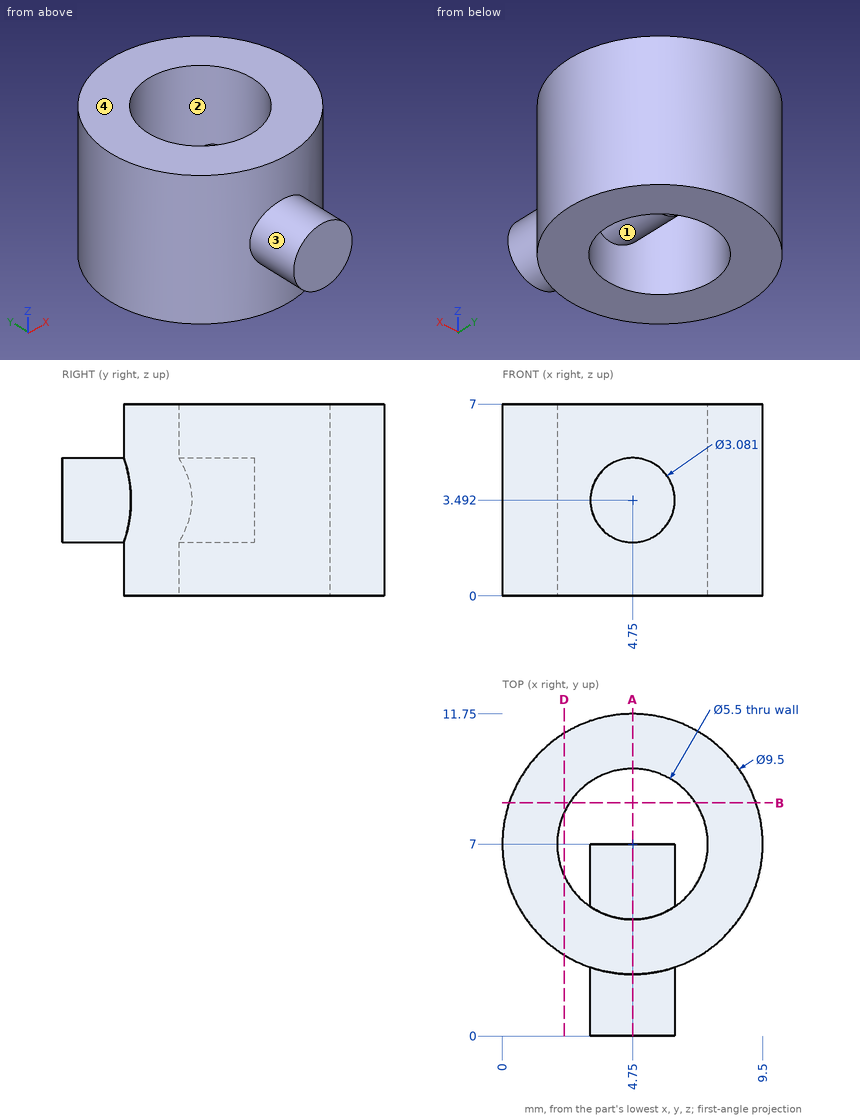
Answer from the drawing. Dimensions are ordinates in mm from the lowest x, y and z of the part. Coordinates: 2 decimals unless noted, no trailing zeros. Order: outer loops, then holes, each group sorted by start corner. A loop starts at its lowest first (then second) coordinate and runs counter-clockwise, first axis right, second up. Notation, with made-up numbers: (-32, 43.5) - (18, 43.5) arc R12 cw to (18, 52.5) - close; hole circle Ø10 at (52, 81.5). An arc over 180 degrees is marked (long way). Put each result on its own line as item: value. Start each with the question number.
1) Find section A-A (x = 4.75). Give the vertices of the cut face in (y, z).
2) Find the intervals of material crossed by line 1 (Y direction, x = 4.75, z = 2.25); line 2 (Y direction, x = 4.75, z = 1.5); line 3 (X direction, y = 6.25, z = 3.5) (1 decimal), in increasing order. Write a range as from..to.
3) Find section B-B (y = 8.5). Give the vertices of the cut face in (x, z) (1 decimal).
4) For a pull along X with two mould halves and no side action, classify the marked faces 1, 2, 3 and 4 as released by +X, released by -X, zero draft, split by the parting line, or undercut.
5) Find section D-D (x = 2.25). Give the vertices of the cut face in (y, z) (1 decimal).
6) A flat-ended cylindrical pin translates along its axis: pin 1 (3.5 mm diameter, centred on x = 4.75, y = 7, fed in from -Z). Find the tip coordinate at first contact, or state that the pin passes through.
Results list:
1. outline: (0, 1.95) - (2.25, 1.95) - (2.25, 0) - (4.25, 0) - (4.25, 1.95) - (7, 1.95) - (7, 5.03) - (4.25, 5.03) - (4.25, 7) - (2.25, 7) - (2.25, 5.03) - (0, 5.03) - close; (9.75, 0) - (11.75, 0) - (11.75, 7) - (9.75, 7) - close
2. line 1: y = 0..7, 9.75..11.75
2. line 2: y = 2.25..4.25, 9.75..11.75
2. line 3: x = 0.1..2.1, 3.2..6.3, 7.4..9.4
3. outline: (0.2, 0) - (2.4, 0) - (2.4, 7) - (0.2, 7) - close; (7.1, 0) - (9.3, 0) - (9.3, 7) - (7.1, 7) - close
4. face 1: undercut
4. face 2: undercut
4. face 3: split by the parting line
4. face 4: zero draft
5. outline: (3, 0) - (5.9, 0) - (5.9, 7) - (3, 7) - close; (8.1, 0) - (11, 0) - (11, 7) - (8.1, 7) - close
6. pin 1: stops at z = 1.95
